from build123d import *

# Parameters (mm, degrees)
BOSS_EXTRU_1_DEPTH      = 6
ENL_V_MAT_EXTRU_1_REACH = 24.65
ESQUISSE2_R             = 3.6
ENL_V_START             = -2.2
ENL_V_MAT_EXTRU_2_DEPTH = 2.2
ESQUISSE6_W             = 2.75
ESQUISSE6_H             = 16
ENL_V_MAT_EXTRU_4_REACH = 37.477
ESQUISSE7_W             = 29.554917854
ESQUISSE7_H             = 36.646442603


with BuildPart() as part:
    # Esquisse1 → Boss.-Extru.1 (new body)
    with BuildSketch(Plane.XY):
        with BuildLine():
            Line((0, 6), (21, 4))
            Line((21, 4), (21, -4))
            Line((21, -4), (0, -6))
            ThreePointArc((0, -6), (-6, 0), (0, 6))
        make_face()
    extrude(amount=BOSS_EXTRU_1_DEPTH)

    # Esquisse2 → Enl_v. mat.-Extru.1 (cut, up to next)
    with BuildSketch(Plane(origin=(0, 0, 0), x_dir=(-1, 0, 0), z_dir=(0, 0, -1)), mode=Mode.PRIVATE) as enl_v_mat_extru_1_sk1:
        Circle(ESQUISSE2_R)
    enl_v_mat_extru_1_tool1 = extrude(enl_v_mat_extru_1_sk1.sketch, amount=-ENL_V_MAT_EXTRU_1_REACH, mode=Mode.PRIVATE) & part.part
    add(enl_v_mat_extru_1_tool1.solids().sort_by_distance((0, 0, 0))[0], mode=Mode.SUBTRACT)

    # Esquisse3 → Enl_v. mat.-Extru.2 (cut)
    with BuildSketch(Plane.XY.offset(6).offset(ENL_V_START)):
        with BuildLine():
            Line((0, 3.6), (16, 2.1))
            ThreePointArc((16, 2.1), (18.1, 0), (16, -2.1))
            Line((16, -2.1), (0, -3.6))
            ThreePointArc((0, -3.6), (-3.6, 0), (0, 3.6))
        make_face()
    extrude(amount=ENL_V_MAT_EXTRU_2_DEPTH, mode=Mode.SUBTRACT)

    # Esquisse6 → R_volution1 (revolve)
    with BuildSketch(Plane.XY.offset(3), mode=Mode.PRIVATE) as r_volution1_sk:
        with Locations((19.625, 1)):
            Rectangle(ESQUISSE6_W, ESQUISSE6_H)
    revolve(r_volution1_sk.sketch.rotate(Axis((25.5, 9, 3), (0, -1, 0)), 90), axis=Axis((25.5, 9, 3), (0, -1, 0)))

    # Esquisse7 → Enl_v. mat.-Extru.4 (cut, up to next)
    with BuildSketch(Plane(origin=(0, 0, 0), x_dir=(-1, 0, 0), z_dir=(0, 0, -1)), mode=Mode.PRIVATE) as enl_v_mat_extru_4_sk1:
        with Locations((-30.387795564, 1.156001867)):
            Rectangle(ESQUISSE7_W, ESQUISSE7_H)
    enl_v_mat_extru_4_tool1 = extrude(enl_v_mat_extru_4_sk1.sketch, amount=ENL_V_MAT_EXTRU_4_REACH, mode=Mode.PRIVATE) & part.part
    add(enl_v_mat_extru_4_tool1.solids().sort_by_distance((30.387796, 1.156002, 0))[0], mode=Mode.SUBTRACT)


solid = part.part
Geometry: final body of the model. Coordinates: model frame, mm. A direction names the side the tool comes from. Round coordinates to 2 decimals unless told otherwise and drop trailing zeros. Order: outer loops, then holes, each group sorted by start corner. A loop starts at its lowest first (then second) coordinate and runs counter-clockwise, first axis right, second up. Notation, with made-up numbers: (-17.75, -25) -> (8.25, -25) arc R18 ccw to (8.25, 7) -> close; hole circle Ø1 at (-26.5, 86.5). An arc over 180 degrees is marked (long way). Put each result on its own line as item: value. Start each with the question number.
Q1. Reachability of faces 4 (the flat face through (7, -4, 6)), 5 (the cylindrical face through (-6, 0, 3)), 6 (the flat face through (8.23, 2.83, 4.88)) from +Z, -Z, +X, -X, +Y, -Y: full face, straight path, thin tool, end or side. Return the list, or none.
Q2. Section C-C on z = 6.75. Return the cut outline in (x, y).
Q3. Line query: probe 1 along Y at (x, z) = (0, 4.25); probe 2 along X at (y, z) = (-0.75, 3.25); probe 3 along X at (y, z) = (0.5, 1). Output: solid intervals per line, ascending.
Q4. First-contact query: pin 1 (1 mm diameter, centred on x = 23.5, z = 6, fed in from +Y); pin 2 (5.5 mm diameter, centred on x = 8.5, y = -1, fed in from +Z). Flat tips, straight axial feed; report the tip coordinate or a pass-through.
Q5. Pull-direction query (Y, two-part tool) for faces 1 (the flat face through (11, -1, 0)), 2 (the flat face through (10, 0, 3.8)), 3 (the flat face through (9.582, -5.087, 2.958)); classes: +Y half, -Y half, draft (parallel to the pull), parting line (faces both ways), or undercut.
Q6. Section D-D on x = 5.5. Return the cut outline in (y, z).
Q7. Section A-A on z = 2. Return the cut outline in (x, y).
Q8. Section B-B on y = 0. Return the cut outline in (x, z).
Ans:
1. face 4: +Z, -X, +Y, -Y
1. face 5: +Z, -Z, -X
1. face 6: +Z
2. outline: (19.3, -7) -> (23.01, -7) -> (23.01, 9) -> (19.3, 9) -> close; (27.99, -7) -> (31.7, -7) -> (31.7, 9) -> (27.99, 9) -> close
3. probe 1: y = -6 to -3.6, 3.6 to 6
3. probe 2: x = -5.95 to -3.52, 3.52 to 21.01, 29.99 to 32.75
3. probe 3: x = -5.98 to -3.57, 3.57 to 21.47, 29.53 to 32.47
4. pin 1: passes through
4. pin 2: stops at z = 6
5. face 1: draft
5. face 2: undercut
5. face 3: -Y half
6. outline: (-5.48, 0) -> (5.48, 0) -> (5.48, 6) -> (3.08, 6) -> (3.08, 3.8) -> (-3.08, 3.8) -> (-3.08, 6) -> (-5.48, 6) -> close
7. outline: (0, -6) -> (18.32, -4.26) -> (18.32, -7) -> (21.11, -7) -> (21.11, 9) -> (18.32, 9) -> (18.32, 4.26) -> (0, 6) arc R6 ccw to start; (29.89, -7) -> (32.68, -7) -> (32.68, 9) -> (29.89, 9) -> close; hole circle Ø7.2 at (0, 0)
8. outline: (-6, 0) -> (-3.6, 0) -> (-3.6, 6) -> (-6, 6) -> close; (3.6, 0) -> (22.15, 0) arc R4.5 cw (long way) to (28.85, 0) -> (32.1, 0) arc R7.25 ccw to (18.9, 6) -> (18.1, 6) -> (18.1, 3.8) -> (3.6, 3.8) -> close
